Check sheet for the drawn part. Datum: minimum x, y, z corner. Units: mm. A direction names the side the tool comes from. Give positions to 0.01 mm unless a question says otherwise; leave off trailing zeros. Write each loop counter-clockwise with the first axis right and the second up, starting at its lowest first coordinate (ties: lowest second). Pieces come first, ordered by that corner, then holes. Notation, with made-up numbers: (-28.75, -6) -> (13.25, -6) arc R29 cw to (13.25, 28) -> close; hole circle Ø9 at (21, -2). An arc over 180 degrees is marked (long way). Write item = value, one per line. Start each with the question number.
1. Cross-section at C-C, the plane x = 18. Record the cut outline in (y, z) (1 decimal).
2. Cross-section at A-A, the plane z = 110.49. State how many separate pieces and enclosed holes the cut face has, plus the area to 3 significant figures.
3. Cross-section at D-D, the plane y = 15.25. Record the cut outline in (x, z) (1 decimal).
4. Depth check by flat-ended pin: P1, Ø3.5, axis at x = 45, y = 1, coming from the -Z side; P2, Ø1.5, axis at x = 39, z = 62.5, coming from the +Y side (1 decimal); P3, Ø10, axis at y = 5.5, z = 23.5, coming from the -X side. Enter the tip coordinate at first touch or a pass-through.
5. Set-up check for the marked faces 1 and 2: record each of +Z, -Z, +X, -X, +Y, -Y from which the full face is reachable in a straight line by a thin tool's end or side.
6. Thickness scan on line 1 along Y through (x, z) = (34.5, 95.5) (1 decimal); line 2 along Z through (x, y) = (43.5, 2.25). Record the ranges inside material, lowest first.
7. Cross-section at B-B, the plane x = 6. Record the cut outline in (y, z) (1 decimal).
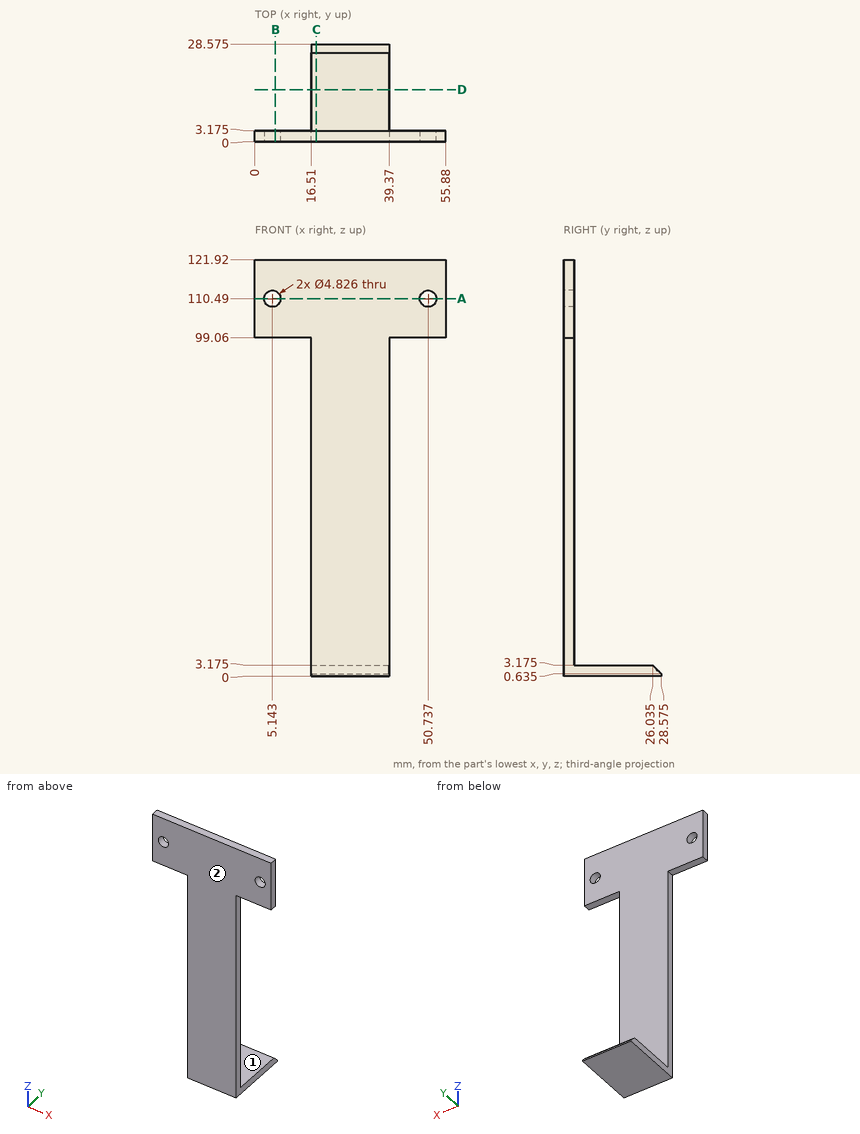
Answers:
q1.outline = (0, 0) -> (28.6, 0) -> (28.6, 0.6) -> (26, 3.2) -> (3.2, 3.2) -> (3.2, 121.9) -> (0, 121.9) -> close
q2.separate_pieces = 3
q2.enclosed_holes = 0
q2.area = 147 mm^2
q3.outline = (16.5, 0) -> (39.4, 0) -> (39.4, 3.2) -> (16.5, 3.2) -> close
q4.P1 = 99.06
q4.P2 = 3.2
q4.P3 = 16.51
q5.face_1 = +Z, +X, -X, +Y
q5.face_2 = +Z, -Z, +X, -X, -Y
q6.line_1 = 0 to 3.2
q6.line_2 = 99.06 to 121.92
q7.outline = (0, 99.1) -> (3.2, 99.1) -> (3.2, 108.2) -> (0, 108.2) -> close; (0, 112.7) -> (3.2, 112.7) -> (3.2, 121.9) -> (0, 121.9) -> close
